Geometry: see drawing. Coordinates: mm, zero at the bounding-box minimum. A direction names the side the tool comes from. Give positions to 0.01 mm unless a question says otherwise; leave off trailing zeros. Write each loop counter-clockwise with the first axis right and the second up, starting at its lowest first coordinate (ties: lowest second). Pieces come first, ordered by that corner, then holes. Notation, with made-up numbers: M 49,7 L 92,7 A23 ccw 92,38 Z; hole C 87,31 d4. An arc over 180 degrees is marked long. Use CSV: the item, a comma, the result in double quotes. Start each with the question number.
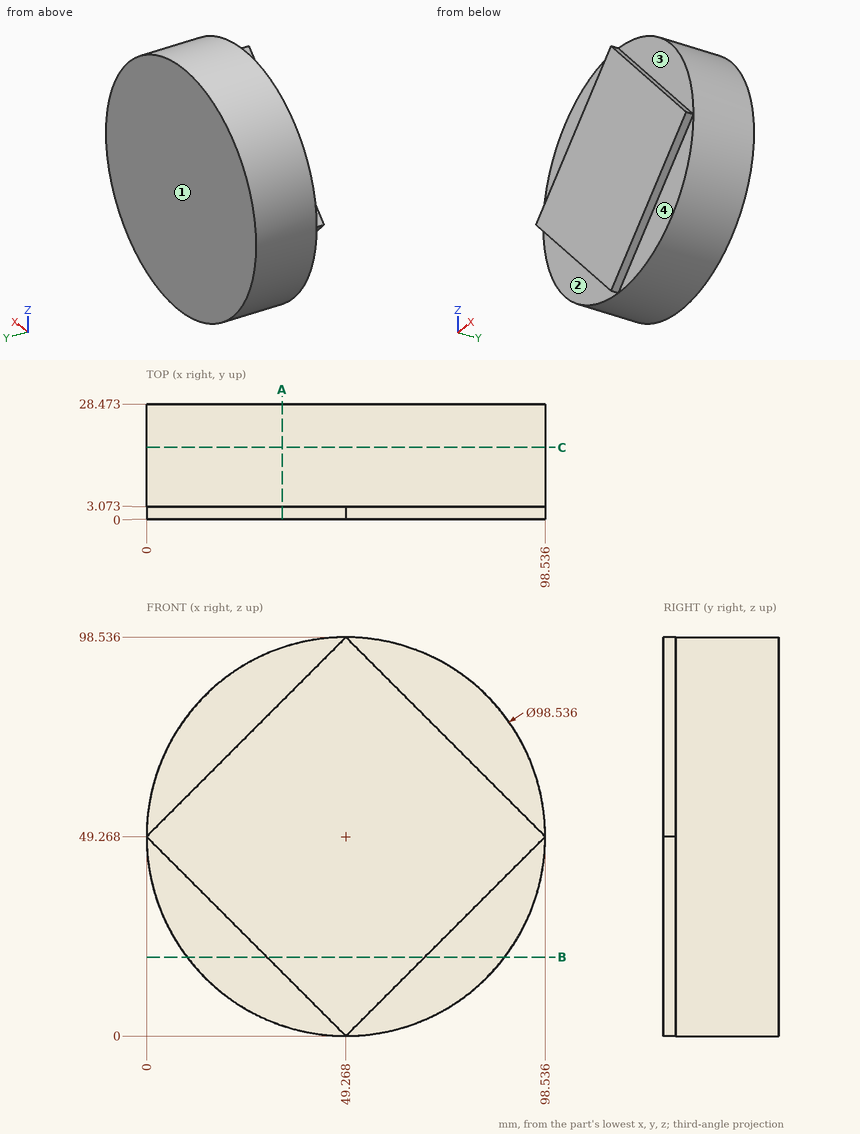
1. Line query: probe 1 along Y at (x, z) = (39.5, 92.5); probe 2 along Z at (x, y) = (50, 5) (1 decimal); probe 3 along Z at (x, y) = (16, 11) (1 decimal). Output: solid intervals per line, ascending.
2. Section B-B on z = 19.5. Return loops of the section in (x, y) (1 decimal), then the cut area to 3 significant figures.
3. First-contact query: pin 1 (5 mm diameter, centred on x = 64, y = 10.5, fed in from -Z); pin 2 (10 mm diameter, centred on x = 26, y = 10.5, fed in from -Z); pin 3 (1.5 mm diameter, centred on x = 84, y = 7, fed in from -Z) (1 decimal). Flat tips, straight axial feed; report the tip coordinate or a pass-through.
4. Access query for the marked faces 1, 2, 3 and 4. Directions: +Z, -Z, +X, -X, +Y, -Y. A direction counts if a zero-diameter tool reaches every point of the face in a straight line with its end or side. Return the directions, or none.
5. Section C-C on y = 17.75. Return loops of the section in (x, z) (1 decimal).
6. Section A-A on x = 33.5. Return loops of the section in (y, z) (1 decimal).
Resolved:
1,probe 1,"y = 3.07 to 28.47"
1,probe 2,"z = 0 to 98.5"
1,probe 3,"z = 12.9 to 85.6"
2,outline,"M 10,3.1 L 29.8,3.1 L 29.8,0 L 68.8,0 L 68.8,3.1 L 88.5,3.1 L 88.5,28.5 L 10,28.5 Z"
2,area,"2,110 mm2"
3,pin 1,"stops at z = 1.54"
3,pin 2,"stops at z = 3.51"
3,pin 3,"stops at z = 13.6"
4,face 1,"+Z, -Z, +X, -X, +Y"
4,face 2,"-Z, -X, -Y"
4,face 3,"+Z, +X, -Y"
4,face 4,"-Z, +X, -Y"
5,outline,"C 49.3,49.3 d98.5"
6,outline,"M 0,15.8 L 3.1,15.8 L 3.1,2.6 L 28.5,2.6 L 28.5,95.9 L 3.1,95.9 L 3.1,82.8 L 0,82.8 Z"
